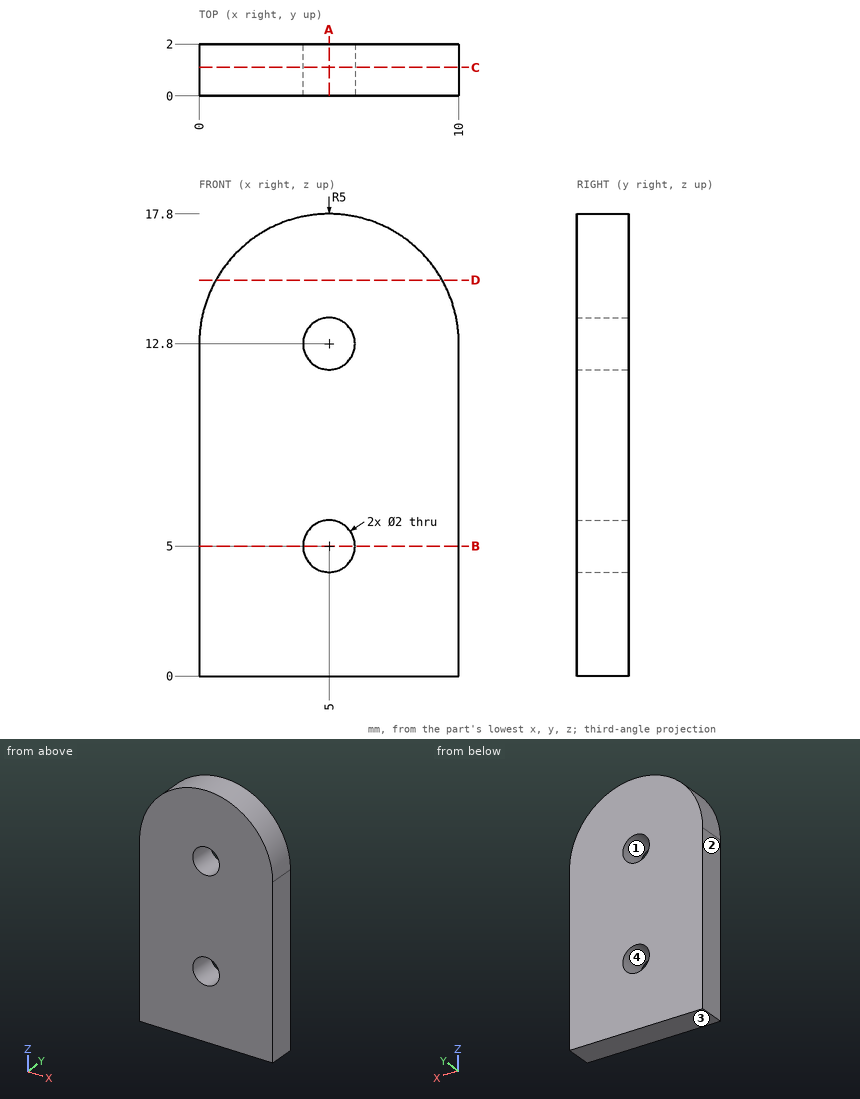
Print and shaded views of the part. All mm, measured from the part's lowest x, y and z. Round coordinates to 2 decimals unless told otherwise and drop trailing zeros. Loops run counter-clockwise (first coordinate to the right, second up) from the corner with the lowest first, then second, coordinate; pieces in that order, holes last. Notation, with made-up numbers: (29, -2) -> (80, -2) arc R20 ccw to (80, 6) -> close; hole circle Ø5 at (38, -7.75). An arc over 180 degrees is marked (long way). Use CSV: the item, a comma, the result in double quotes. Start each with the question number.
1) Cut at C-C, the plane y = 1.1. Write the cut outline in (x, z).
2) Pull direction X, two halves, no side cores. Call the marked faces 1, 2, 3 and 4: +X half, -X half, draft (parallel to the pull), parting line (faces both ways), or undercut.
3) Cut at D-D, the plane z = 15.25. Write the cut outline in (x, y).
4) Cut at B-B, the plane z = 5. Write the cut outline in (x, y), plus the area to 3 significant figures.
5) Wall check: L1, parallel to Z at x = 5, y = 0.7; L2, parallel to X at y = 0.7, z = 12.25; L3, parallel to Z at x = 8, y = 0.4. Give the ranges that are in metal, low to high. Write a range as [from, to].
6) Cut at A-A, the plane x = 5. Write the cut outline in (y, z), plus the area to 3 significant figures.
Determined:
1,outline,"(0, 0) -> (10, 0) -> (10, 12.8) arc R5 ccw to (0, 12.8) -> close; hole circle Ø2 at (5, 5); hole circle Ø2 at (5, 12.8)"
2,face 1,"undercut"
2,face 2,"-X half"
2,face 3,"draft"
2,face 4,"undercut"
3,outline,"(0.64, 0) -> (9.36, 0) -> (9.36, 2) -> (0.64, 2) -> close"
4,outline,"(0, 0) -> (4, 0) -> (4, 2) -> (0, 2) -> close; (6, 0) -> (10, 0) -> (10, 2) -> (6, 2) -> close"
4,area,"16.0 mm2"
5,L1,"z = [0, 4], [6, 11.8], [13.8, 17.8]"
5,L2,"x = [0, 4.16], [5.84, 10]"
5,L3,"z = [0, 16.8]"
6,outline,"(0, 0) -> (2, 0) -> (2, 4) -> (0, 4) -> close; (0, 6) -> (2, 6) -> (2, 11.8) -> (0, 11.8) -> close; (0, 13.8) -> (2, 13.8) -> (2, 17.8) -> (0, 17.8) -> close"
6,area,"27.6 mm2"
